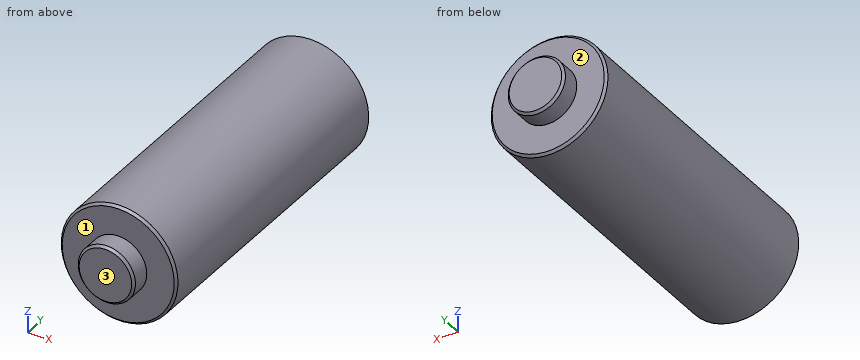
from build123d import *

# Parameters (mm, degrees)
SKETCH1_R           = 2.45
BOSS_EXTRUDE1_DEPTH = 30
CHAMFER1_SIZE       = 0.2
SKETCH2_R           = 5
BOSS_EXTRUDE2_DEPTH = 13.25
CHAMFER2_SIZE       = 0.2


with BuildPart() as part:
    # Sketch1 → Boss-Extrude1 (new body)
    with BuildSketch(Plane(origin=(0, 0, 0), x_dir=(1, 0, 0), z_dir=(0, 1, 0))):
        with Locations(Location((0, 0, 0), (0, 0, 270))):
            Circle(SKETCH1_R)
    extrude(amount=BOSS_EXTRUDE1_DEPTH)

    # Chamfer1
    chamfer1_edges = [part.edges().sort_by_distance(p)[0] for p in [
        (0, 0, -2.45),
        (0, 30, -2.45),
    ]]
    chamfer(chamfer1_edges, length=CHAMFER1_SIZE)

    # Sketch2 → Boss-Extrude2 (add, symmetric)
    with BuildSketch(Plane(origin=(0, 15, 0), x_dir=(1, 0, 0), z_dir=(0, 1, 0))):
        with Locations(Location((0, 0, 0), (0, 0, 270))):
            Circle(SKETCH2_R)
    extrude(amount=BOSS_EXTRUDE2_DEPTH, both=True)

    # Chamfer2
    chamfer2_edges = [part.edges().sort_by_distance(p)[0] for p in [
        (0, 1.75, -5),
        (0, 28.25, -5),
    ]]
    chamfer(chamfer2_edges, length=CHAMFER2_SIZE)


solid = part.part
For this review, take the finished solid that the model builds, in its own axes (mm). Face numbers are marked on the shaded views. A direction names the side the tool comes from. Round coordinates to 2 decimals unless told otherwise and drop trailing zeros. Loops run counter-clockwise (first coordinate to the right, second up) from the corner with the lowest first, then second, coordinate; pieces in that order, holes last. Notation, with made-up numbers: (-31, 83) - (-21, 83) arc R23 cw to (-21, 104) - close; hole circle Ø6 at (-12, -15.75). An arc over 180 degrees is marked (long way). One line per item, written item: value. Start each with the question number.
Item 1: Take a section at A-A (x = 0). Give the boundary of the cut face in (y, z), plus the area to 3 significant figures.
Item 2: Clearance check with flat-ended pins moving along their axes: pin 1 Ø1 at (x, y) = (2, 4) entering from -Z; pin 2 Ø1.5 at (x, z) = (3, 3.5) entering from -Y. State where each tip first meets the part, or that it passes through.
Item 3: For the marked faces 1, 2 and 3, list the 3-axis set-ups (+Z, -Z, +X, -X, +Y, -Y) from which the entire face can be reached by the end or side of a thin tool; tool diameter is ignored.
Item 4: For L1, parallel to Y at x = 3.5, z = -3; L2, parallel to X at y = 15.25, z = 0.25; L3, parallel to X at y = 7.25, z = 1.75, list the stretches that pass through material, from the lowest coordinate up.
Item 5: Take a section at C-C (y = 8.5). Give the boundary of the cut face in (x, z), plus the area to 3 significant figures.
Item 6: Take a section at B-B (z = 0). Give the boundary of the cut face in (x, y).
Answer below:
1. outline: (0, -2.25) - (0.2, -2.45) - (1.75, -2.45) - (1.75, -4.8) - (1.95, -5) - (28.05, -5) - (28.25, -4.8) - (28.25, -2.45) - (29.8, -2.45) - (30, -2.25) - (30, 2.25) - (29.8, 2.45) - (28.25, 2.45) - (28.25, 4.8) - (28.05, 5) - (1.95, 5) - (1.75, 4.8) - (1.75, 2.45) - (0.2, 2.45) - (0, 2.25) - close
1. area: 282 mm2
2. pin 1: stops at z = -4.77
2. pin 2: stops at y = 1.75
3. face 1: -Y
3. face 2: +Y
3. face 3: +Z, -Z, +X, -X, -Y
4. L1: y = 1.75 to 28.25
4. L2: x = -4.99 to 4.99
4. L3: x = -4.68 to 4.68
5. outline: circle Ø10 at (0, 0)
5. area: 78.5 mm2
6. outline: (-5, 1.95) - (-4.8, 1.75) - (-2.45, 1.75) - (-2.45, 0.2) - (-2.25, 0) - (2.25, 0) - (2.45, 0.2) - (2.45, 1.75) - (4.8, 1.75) - (5, 1.95) - (5, 28.05) - (4.8, 28.25) - (2.45, 28.25) - (2.45, 29.8) - (2.25, 30) - (-2.25, 30) - (-2.45, 29.8) - (-2.45, 28.25) - (-4.8, 28.25) - (-5, 28.05) - close
